from build123d import *

# Parameters (mm, degrees)
F0_W     = 97
F0_H     = 126
F0_R     = 2
F0_R_2   = 13
F1_DEPTH = 3
F4_R     = 3
F5_R     = 3
F6_R     = 2.99999


# Not quite as in the source:
# - a fillet or chamfer that OpenCascade refuses, or shapes differently, is made with other operations: its cross-section is extruded or revolved along the edge and cut away or added
# - a fillet or chamfer is up to 0.001 mm smaller than in the source, because OpenCascade refuses the exact size


with BuildPart() as f1:
    # F0 (on Top) → F1 (new body)
    with BuildSketch(Plane.XY):
        Rectangle(F0_W, F0_H)
        with Locations((-42, -56.5)):
            Circle(F0_R, mode=Mode.SUBTRACT)
        with Locations((-22.5, -27.884999302)):
            Circle(F0_R_2, mode=Mode.SUBTRACT)
        with Locations((42, -56.5)):
            Circle(F0_R, mode=Mode.SUBTRACT)
        with Locations((22.5, -27.8849992901)):
            Circle(F0_R_2, mode=Mode.SUBTRACT)
        with Locations((-42, 56.5)):
            Circle(F0_R, mode=Mode.SUBTRACT)
        with Locations((42, 56.5)):
            Circle(F0_R, mode=Mode.SUBTRACT)
    extrude(amount=F1_DEPTH)

    # F2: fillet of radius 5 on 1 edges, made by hand

    # F2_s1 → F2_t2 (revolve, cut)
    with BuildSketch(Plane.XZ.offset(27.884999302)):
        with BuildLine():
            ThreePointArc((-9.5, 3), (-7.6560370926, 0.8166998673), (-4.917424305, 0))
            Line((-4.917424305, 0), (-9.5, 0))
            Line((-9.5, 0), (-9.5, 3))
        make_face()
    revolve(axis=Axis((-22.5, -27.884999302, 0), (0, 0, 1)), mode=Mode.SUBTRACT)

    # F3: fillet of radius 5 on 1 edges, made by hand

    # F3_s1 → F3_t2 (revolve, cut)
    with BuildSketch(Plane.XZ.offset(27.8849992901)):
        with BuildLine():
            ThreePointArc((40.082575695, 0), (37.3439629074, 0.8166998673), (35.5, 3))
            Line((35.5, 3), (35.5, 0))
            Line((35.5, 0), (40.082575695, 0))
        make_face()
    revolve(axis=Axis((22.5, -27.8849992901, 0), (0, 0, 1)), mode=Mode.SUBTRACT)

    # F4
    f4_edges = [f1.edges().sort_by_distance(p)[0] for p in [
        (48.5, -63, 1.5),
        (-48.5, -63, 1.5),
    ]]
    fillet(f4_edges, radius=F4_R)

    # F5
    f5_edges = [f1.edges().sort_by_distance(p)[0] for p in [
        (48.5, 63, 1.5),
        (-48.5, 63, 1.5),
    ]]
    fillet(f5_edges, radius=F5_R)

    # F6 (radius 3 in the source; OpenCascade refuses exactly that, so slightly less here)
    f6_edges = [f1.edges().sort_by_distance(p)[0] for p in [
        (0, -63, 3),
        (47.62132, -62.12132, 3),
        (48.5, 0, 3),
        (47.62132, 62.12132, 3),
        (0, 63, 3),
        (-47.62132, 62.12132, 3),
        (-48.5, 0, 3),
        (-47.62132, -62.12132, 3),
    ]]
    fillet(f6_edges, radius=F6_R)


solid = f1.part
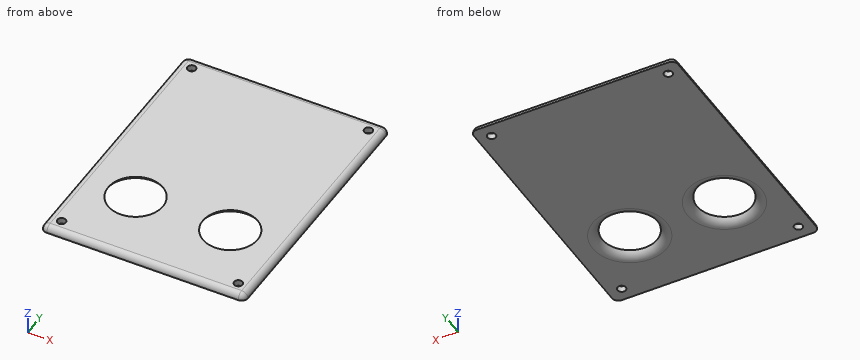
The listing builds one solid part. Answer for the finished solid, in the listing's coordinates (mm). Give positions to 0.01 mm unless a question says otherwise; leave off trailing zeros. One line per question, with ' | ' between items. Start each with the question number.
1. Section A-A, the plane x = -42 is taken. Count the separate pieces of the cut face and the enclosed holes in it, then the cut area to 3 significant figures.
2. Given P1, Ø3.5, axis at x = -42, y = 56.5, coming from the +Z side; P2, Ø1.5, axis at y = -34, z = 1, coming from the +X side, each flat-ended and moving along its own axis, determine where each tip first touches the part or whether it passes through.
3. Straight lines are drawn through the part: line 1 (Y direction, x = 42, z = 1.55); line 2 (X direction, y = -20.5, z = 2.15); line 3 (Y direction, x = 42, z = 1.05). For each, find the intervals that lie inside material, in ascending order.
Result:
1) separate pieces: 3 | enclosed holes: 0 | area: 350 mm2
2) P1: passes through | P2: stops at x = 48.49
3) line 1: y = -62.57 to -58.5, -54.5 to 54.5, 58.5 to 62.57 | line 2: x = -47.59 to -33.77, -11.23 to 11.23, 33.77 to 47.59 | line 3: y = -62.81 to -58.5, -54.5 to 54.5, 58.5 to 62.81
